Geometry: see drawing. Coordinates: mm, zero at the bounding-box minimum. Give positions to 0.01 mm unless a question says otherwise; leave off trailing zeros. Order: outer loops, then holes, each group sorted by start corner. A loop starts at its lowest first (then second) coordinate and runs counter-clockwise, first axis right, second up. Notation, with made-up numbers: (-35, 78) - (-31, 78) arc R30 cw to (-31, 109) - close; hole circle Ø3 at (-8, -24). An arc over 180 degrees is marked (long way). One line per item, written item: value.
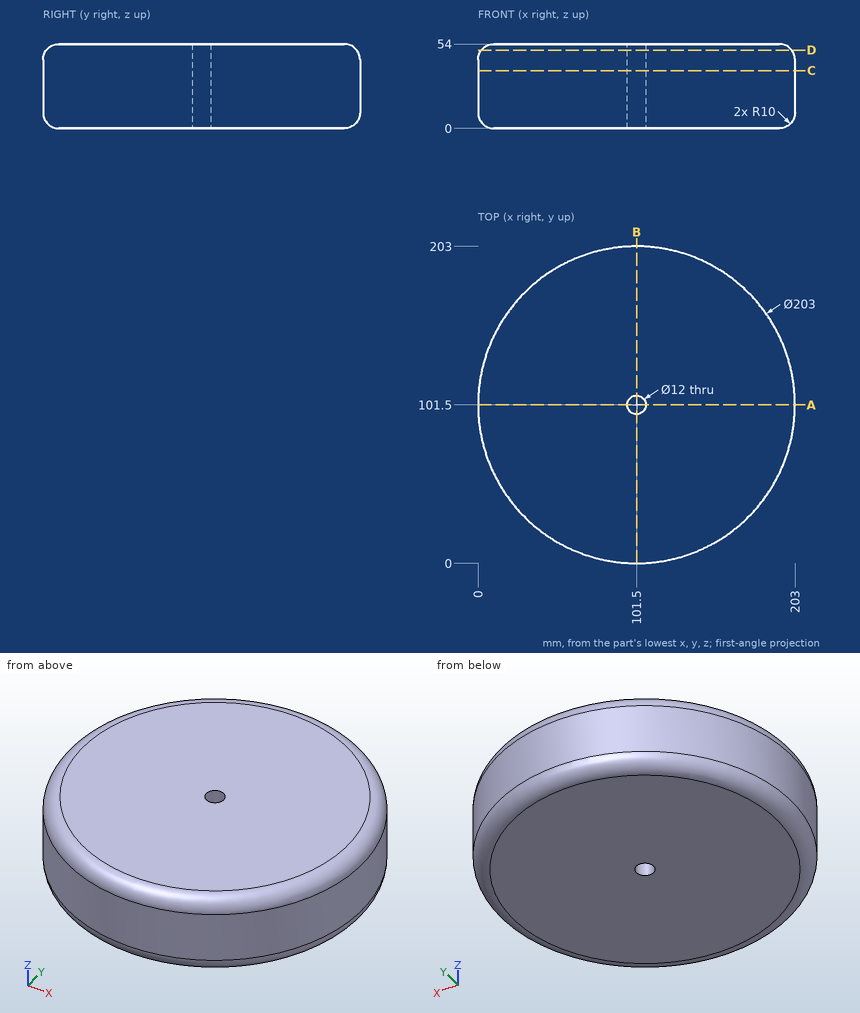
1) Section C-C, the plane z = 37. Return loops of the section in (x, y), then the cut area to 3 significant figures.
Answers below:
outline: circle Ø203 at (101.5, 101.5); hole circle Ø12 at (101.5, 101.5)
area: 32,300 mm^2
2) First-contact query: pin 1 (3 mm diameter, centred on y = 80.5, z = 31.5, fed in from +X); pin 2 (8 mm diameter, centred on x = 50.5, z = 22.5, fed in from -Y); pin 3 (5 mm diameter, centred on y = 164, z = 45, fed in from +X). Flat tips, straight axial feed; report the tip coordinate or a pass-through.
Answers below:
pin 1: x = 201.11
pin 2: y = 11.54
pin 3: x = 183.32
3) Section D-D, the plane z = 50. Return loops of the section in (x, y), then the cut area to 3 significant figures.
Answers below:
outline: circle Ø199 at (101.5, 101.5); hole circle Ø12 at (101.5, 101.5)
area: 31,000 mm^2
4) Material intervals for line 1 along Y through (x, z) = (101, 19); line 2 along Y through (x, z) = (103, 6), sorted ascending.
Answers below:
line 1: 0 to 95.52, 107.48 to 203
line 2: 0.85 to 95.69, 107.31 to 202.15
5) Section A-A, the plane y = 101.5. Return loops of the section in (x, z), then the cut area to 3 significant figures.
Answers below:
outline: (0, 10) arc R10 ccw to (10, 0) - (95.5, 0) - (95.5, 54) - (10, 54) arc R10 ccw to (0, 44) - close; (107.5, 0) - (193, 0) arc R10 ccw to (203, 10) - (203, 44) arc R10 ccw to (193, 54) - (107.5, 54) - close
area: 10,200 mm^2
